Could you check a few things on this model? Use its own coordinates, in mm. Face numbers are marked on the shaded views. A direction names the side the tool comes from. Coordinates: 2 decimals unless noted, no trailing zeros. Loops run counter-clockwise (first coordinate to the right, second up) from the corner with the lowest first, then second, coordinate; pieces in that order, holes last.
1) Thinking about a two-plate mould opening in Z: for the marked faces 1, 2 and 3, which applies, released by +Z, released by -Z, zero draft, split by the parting line, or undercut?
2) If I drill on line 1 along Z through (x, y) = (0, 6.3); line 2 along Z through (x, y) = (3.75, 4.75), over which ranges is the centre line in solid material (lowest first)?
3) Will these pins go through, and if not, where does the flat tip stop? P1, Ø3, axis at y = 6.5, z = 0.5, coming from the -X side; P2, Ø1, axis at x = 2.5, y = 4, coming from the -Z side; P3, Ø4, axis at x = 3, y = 2, coming from the +Z side.
4) For the marked faces 4, 5, 6 and 7, which set-ups out of +Z, -Z, +X, -X, +Y, -Y let a thin tool reach every point of the face, with its end or its side?
5) Imagine slicing it at A-A on y = 7. Please give me the cut outline in (x, z).
```python
from build123d import *

# Parameters (mm, degrees)
BOSS_EXTRUDE1_DEPTH = 3
CHAMFER1_SIZE       = 1
BOSS_EXTRUDE2_DEPTH = 1


with BuildPart() as part:
    # Sketch1 → Boss-Extrude1 (new body)
    with BuildSketch(Plane(origin=(0, 0, 0), x_dir=(1, 0, 0), z_dir=(0, 1, 0))):
        with BuildLine():
            Line((8.307086349, 9.9), (0, 9.9))
            ThreePointArc((0, 9.9), (-6.363597336, -7.583839987), (9.749596755, 1.719116959))
            Line((9.749596755, 1.719116959), (9.312150139, 4.2))
            Line((9.312150139, 4.2), (3.853569774, 4.2))
            ThreePointArc((3.853569774, 4.2), (5.218014359, 2.293976056), (5.7, 0))
            ThreePointArc((5.7, 0), (-4.030508653, -4.030508653), (0, 5.7))
            Line((0, 5.7), (9.047659668, 5.7))
            Line((9.047659668, 5.7), (8.307086349, 9.9))
        make_face()
    extrude(amount=BOSS_EXTRUDE1_DEPTH)

    # Chamfer1
    chamfer1_edges = [part.edges().sort_by_distance(p)[0] for p in [
        (-6.363597336, 3, 7.583839987),
        (9.530873447, 3, -2.959558479),
        (8.677373008, 3, -7.8),
        (4.153543174, 3, -9.9),
    ]]
    chamfer(chamfer1_edges, length=CHAMFER1_SIZE)

    # Sketch3 → Boss-Extrude2 (add)
    with BuildSketch(Plane(origin=(0, 3, 0), x_dir=(1, 0, 0), z_dir=(0, 1, 0))):
        with BuildLine():
            Line((0, 5.7), (8.032233056, 5.7))
            Line((8.032233056, 5.7), (7.467986717, 8.9))
            Line((7.467986717, 8.9), (0, 8.9))
            ThreePointArc((0, 8.9), (-5.720809726, -6.817795544), (8.764789002, 1.545468781))
            Line((8.764789002, 1.545468781), (8.296723527, 4.2))
            Line((8.296723527, 4.2), (3.853569774, 4.2))
            ThreePointArc((3.853569774, 4.2), (-2.067607313, -5.311779363), (0, 5.7))
        make_face()
    extrude(amount=BOSS_EXTRUDE2_DEPTH)

    # Mirror1: part across plane


with BuildPart() as part_1:
    add(part.part)
    add(part.part.mirror(Plane.ZX.offset(4)))


solid = part_1.part
```
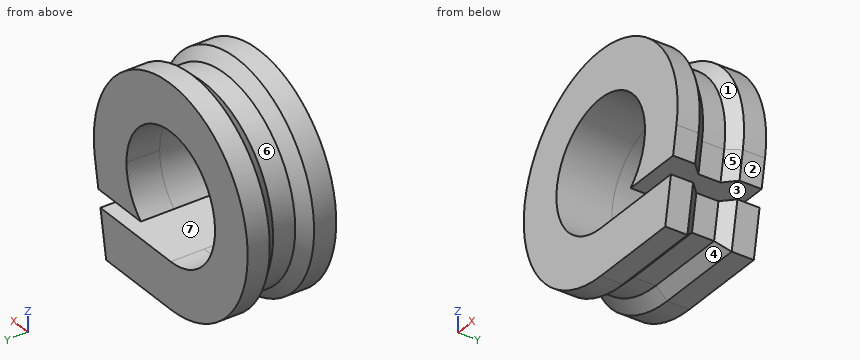
Filled in:
1. face 1: split by the parting line
1. face 2: released by -Z
1. face 3: undercut
2. line 1: z = -9.9 to -5.7, 5.7 to 9.9
2. line 2: z = -8.9 to -5.7, 4.29 to 8.07
3. P1: stops at x = -9.9
3. P2: stops at z = -8.9
3. P3: stops at z = 9.85
4. face 4: -Z, +X, -X
4. face 5: -Z, +X
4. face 6: none
4. face 7: +X, +Y, -Y
5. outline: (0, -9.9) - (8.31, -9.9) - (9.05, -5.7) - (0, -5.7) arc R5.7 cw (long way) to (3.85, -4.2) - (9.31, -4.2) - (9.75, -1.72) arc R9.9 ccw (long way) to start
